Here's how the part is built. I have some questions about the finished solid (model axes, mm). Face numbers are marked on the shaded views. A direction names the side the tool comes from. Give positions to 0.01 mm unless a question says otherwise; leave off trailing zeros. Loops run counter-clockwise (first coordinate to the right, second up) from the corner with the lowest first, then second, coordinate; pieces in that order, holes last. Notation, with made-up numbers: (41, 75) -> (50, 75) arc R12 cw to (50, 85) -> close; hole circle Ø5 at (-35.5, -31.5). An arc over 180 degrees is marked (long way). Answer in a Markdown table with one row per item. Add a question column.
Item 1: If we section it at C-C (z = -13.75): Write out the boundary of the cut face in (x, y).
Item 2: If I drill on line 1 (X direction, y = 11, z = -2); line 2 (Y direction, x = -5.5, z = -1); line 3 (Y direction, x = 16, z = -7.5), over which ranges is the centre line in solid material (lowest first)?
Item 3: If we section it at A-A (x = 0): Write out the boundary of the cut face in (y, z).
Item 4: For P1, Ø8, axis at y = -4.5, z = -1.5, coming from the +X side; P2, Ø4, axis at x = -16.5, z = -2.5, coming from the +Y side; P3, Ø6, axis at y = 5.5, z = -10.5, coming from the -X side, each with a flat end and sliding along its axis, tell me the tip position at first contact or that it passes through.
Item 5: Which directions (+Z, -Z, +X, -X, +Y, -Y) give clear straight access to the entire face, cutting with the end or side of a thin tool? Please do the marked faces 1 and 2.
Item 6: If we section it at B-B (z = 2.25): Write out the boundary of the cut face in (x, y), then the cut area to 3 significant figures.
Item 7: We'd pull the mould along X, two halves only. Please class the marked faces 3, 4, 5 and 6: released by +X, released by -X, zero draft, split by the parting line, or undercut.
```python
from build123d import *

# Parameters (mm, degrees)
F0_R     = 26
F1_DEPTH = 3
F2_DEPTH = 15
F3_SIZE2 = 1.819851
F3_SIZE  = 5


with BuildPart() as f1:
    # F0 (on Top) → F1 (new body)
    with BuildSketch(Plane.XY):
        Circle(F0_R)
        with BuildLine():
            ThreePointArc((3, 22.803509), (17.291616, 15.165751), (23, 0))
            ThreePointArc((23, 0), (22.557855, -4.488117), (21.248418, -8.803678))
            ThreePointArc((21.248418, -8.803678), (19.918584, -11.5), (18.248418, -13.99983))
            ThreePointArc((18.248418, -13.99983), (0, -23), (-18.248418, -13.99983))
            ThreePointArc((-18.248418, -13.99983), (-19.918584, -11.5), (-21.248418, -8.803678))
            ThreePointArc((-21.248418, -8.803678), (-19.918584, 11.5), (-3, 22.803509))
            ThreePointArc((-3, 22.803509), (0, 23), (3, 22.803509))
        make_face(mode=Mode.SUBTRACT)
    extrude(amount=F1_DEPTH)

    # F0 (on Top) → F2 (join)
    with BuildSketch(Plane.XY):
        Circle(F0_R)
        with BuildLine():
            ThreePointArc((3, 22.803509), (17.291616, 15.165751), (23, 0))
            ThreePointArc((23, 0), (22.557855, -4.488117), (21.248418, -8.803678))
            ThreePointArc((21.248418, -8.803678), (19.918584, -11.5), (18.248418, -13.99983))
            ThreePointArc((18.248418, -13.99983), (0, -23), (-18.248418, -13.99983))
            ThreePointArc((-18.248418, -13.99983), (-19.918584, -11.5), (-21.248418, -8.803678))
            ThreePointArc((-21.248418, -8.803678), (-19.918584, 11.5), (-3, 22.803509))
            ThreePointArc((-3, 22.803509), (0, 23), (3, 22.803509))
        make_face(mode=Mode.SUBTRACT)
    extrude(amount=-F2_DEPTH)

    # F3
    f3_edges = [f1.edges().sort_by_distance(p)[0] for p in [
        (-26, 0, -15),
    ]]
    chamfer(f3_edges, length=F3_SIZE, length2=F3_SIZE2)


solid = f1.part
```
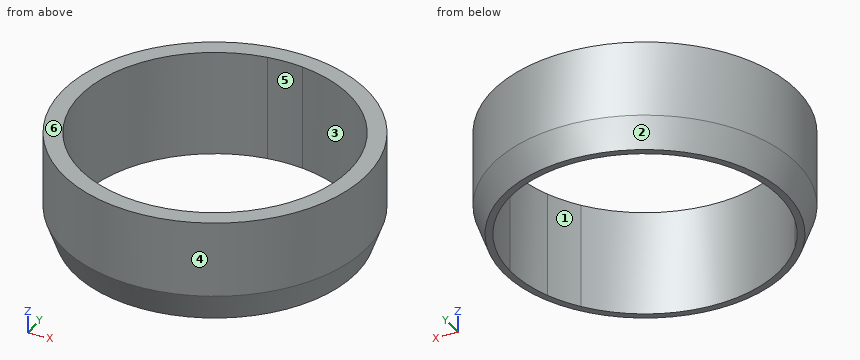
Recorded:
| question | item | result |
|---|---|---|
| 1 | outline | circle Ø49.27 at (0, 0); hole (-21.25, -8.8) arc R23 ccw to (-18.25, -14) arc R23 ccw to (18.25, -14) arc R23 ccw to (21.25, -8.8) arc R23 ccw to (23, 0) arc R23 ccw to (3, 22.8) arc R23 ccw to (-3, 22.8) arc R23 ccw to start |
| 2 | line 1 | x = -23.56 to -20.2, 20.2 to 23.56 |
| 2 | line 2 | y = -25.41 to -22.33, 22.33 to 25.41 |
| 2 | line 3 | y = -20.49 to -16.52, 16.52 to 20.49 |
| 3 | outline | (-26, -10) -> (-24.18, -15) -> (-23, -15) -> (-23, 3) -> (-26, 3) -> close; (23, -15) -> (24.18, -15) -> (26, -10) -> (26, 3) -> (23, 3) -> close |
| 4 | P1 | stops at x = 26 |
| 4 | P2 | stops at y = 21.58 |
| 4 | P3 | stops at x = -25.88 |
| 5 | face 1 | +Z, -Z |
| 5 | face 2 | -Z |
| 6 | outline | circle Ø52 at (0, 0); hole (-21.25, -8.8) arc R23 ccw to (-18.25, -14) arc R23 ccw to (18.25, -14) arc R23 ccw to (21.25, -8.8) arc R23 ccw to (23, 0) arc R23 ccw to (3, 22.8) arc R23 ccw to (-3, 22.8) arc R23 ccw to start |
| 6 | area | 462 mm^2 |
| 7 | face 3 | undercut |
| 7 | face 4 | split by the parting line |
| 7 | face 5 | undercut |
| 7 | face 6 | zero draft |
